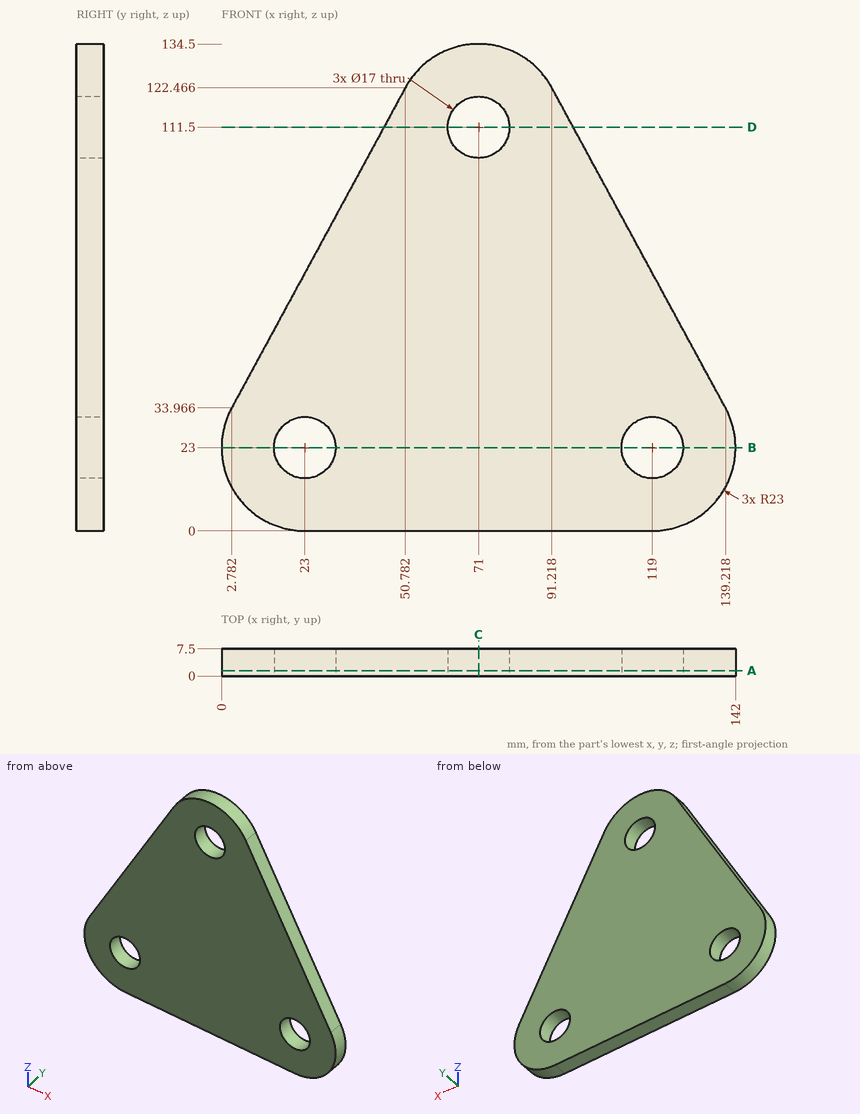
Answer from the drawing. Dimensions are ordinates in mm from the lowest x, y and z of the part. Give positions to 0.01 mm unless a question says otherwise; leave off trailing zeros. Order: outer loops, then holes, each group sorted by start corner. A loop starts at its lowest first (then second) coordinate and runs counter-clockwise, first axis right, second up. Notation, with made-up numbers: (43.5, 58.5) - (100.5, 58.5) arc R25 ccw to (100.5, 94.5) - close; hole circle Ø11 at (-29.75, 49.5). An arc over 180 degrees is marked (long way). One line per item, written item: value. Start each with the question number.
1. Section A-A, the plane y = 1.5 is taken. Write down the section's boundary in (x, z) (1 decimal), then the cut area to 3 significant figures.
2. Section C-C, the plane x = 71 is taken. Write down the section's boundary in (y, z).
3. Section D-D, the plane z = 111.5 is taken. Write down the section's boundary in (x, y) (1 decimal).
4. Section B-B, the plane z = 23 is taken. Write down the section's boundary in (x, y).
5. Consider line 1 (X direction, y = 2.5, z = 23); line 2 (Z direction, x = 71, y = 2.25); line 3 (Z direction, x = 117, y = 4.75) (1 decimal). Determine where each line is inside the solid, lowest interval first.
6. Each of these flat-tipped pins is pushed along its axis until it touches: pin 1 Ø2 at (y, z) = (5, 90.5) entering from +X; pin 2 Ø13.5 at (x, z) = (71, 111.5) entering from +Y; pin 3 Ø1.5 at (y, z) = (4.5, 80.5) entering from +X (1 decimal); pin 4 Ø3 at (x, y) = (112, 3) entering from +Z (1 decimal). Where does it stop, or does it pass through?
Filled sheet:
1. outline: (2.8, 34) arc R23 ccw to (23, 0) - (119, 0) arc R23 ccw to (139.2, 34) - (91.2, 122.5) arc R23 ccw to (50.8, 122.5) - close; hole circle Ø17 at (23, 23); hole circle Ø17 at (71, 111.5); hole circle Ø17 at (119, 23)
1. area: 12,100 mm²
2. outline: (0, 0) - (7.5, 0) - (7.5, 103) - (0, 103) - close; (0, 120) - (7.5, 120) - (7.5, 134.5) - (0, 134.5) - close
3. outline: (44.8, 0) - (62.5, 0) - (62.5, 7.5) - (44.8, 7.5) - close; (79.5, 0) - (97.2, 0) - (97.2, 7.5) - (79.5, 7.5) - close
4. outline: (0, 0) - (14.5, 0) - (14.5, 7.5) - (0, 7.5) - close; (31.5, 0) - (110.5, 0) - (110.5, 7.5) - (31.5, 7.5) - close; (127.5, 0) - (142, 0) - (142, 7.5) - (127.5, 7.5) - close
5. line 1: 0 to 14.5, 31.5 to 110.5, 127.5 to 142
5. line 2: 0 to 103, 120 to 134.5
5. line 3: 0 to 14.7, 31.3 to 74.9
6. pin 1: x = 109.1
6. pin 2: through
6. pin 3: x = 114.4
6. pin 4: z = 86.9
